Design review of the part built by this model. Coordinates are the model's own, in mm. Face numbers are marked on the shaded views. A direction names the side the tool comes from. Give positions to 0.01 mm unless a question says otherwise; leave off trailing zeros. Write each loop counter-clockwise with the first axis right and the second up, starting at its lowest first coordinate (ties: lowest second). Pieces come first, ordered by that corner, then holes.
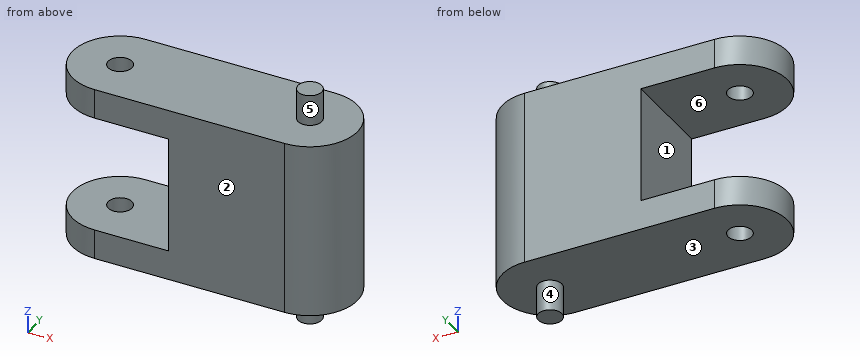
```python
from build123d import *

# Parameters (mm, degrees)
CROQUIS1_R                    = 9.977
SALIENTE_EXTRUIR9_DEPTH       = 148
SALIENTE_EXTRUIR10_DEPTH      = 26
SALIENTE_EXTRUIR10_DEPTH_BACK = 174
CROQUIS8_R                    = 9.977
CROQUIS9_W                    = 114.38894851
CROQUIS9_H                    = 98
CORTAR_EXTRUIR2_DEPTH         = 131


with BuildPart() as part:
    # Croquis1 → Saliente-Extruir9 (new body)
    with BuildSketch(Plane.XY):
        with BuildLine():
            Line((0, 40), (160, 40))
            ThreePointArc((160, 40), (200, 0), (160, -40))
            Line((160, -40), (0, -40))
            ThreePointArc((0, -40), (-40, 0), (0, 40))
        make_face()
        Circle(CROQUIS1_R, mode=Mode.SUBTRACT)
    extrude(amount=SALIENTE_EXTRUIR9_DEPTH)

    # Croquis8 → Saliente-Extruir10 (add, two sides: drawn at the far end of the back side and taken through both)
    with BuildSketch(Plane(origin=(0, 0, 0), x_dir=(-1, 0, 0), z_dir=(0, 0, -1)).offset(-SALIENTE_EXTRUIR10_DEPTH_BACK)):
        with Locations((-160, 0)):
            Circle(CROQUIS8_R)
    extrude(amount=SALIENTE_EXTRUIR10_DEPTH + SALIENTE_EXTRUIR10_DEPTH_BACK)

    # Croquis9 → Cortar-Extruir2 (cut)
    with BuildSketch(Plane(origin=(0, 40, 0), x_dir=(1, 0, 0), z_dir=(0, 1, 0))):
        with Locations((4.810807807, -74)):
            Rectangle(CROQUIS9_W, CROQUIS9_H)
    extrude(amount=-CORTAR_EXTRUIR2_DEPTH, mode=Mode.SUBTRACT)


solid = part.part
```
(1) Tool access review of the marked faces 4, 5 and 6: name each direction out of +Z, -Z, +X, -X, +Y, -Y from which nothing blocks a thin tool from reaching the whole face with its end or side.
Resolved:
face 4: -Z
face 5: +Z
face 6: -X, +Y, -Y
(2) Consider section C-C, the plane x = 79. Give the boundary of the cut face in (y, z), then the cut area to 3 significant figures.
Resolved:
outline: (-40, 0) - (40, 0) - (40, 148) - (-40, 148) - close
area: 11,800 mm2
(3) Mouldability with a two-part tool opening along Z and no side actions: class the marked faces 1, 2 and 3 as pulls with the +Z half, pulls with the -Z half, needs draft (parallel to the pull), parting line crosses it, or undercut.
Resolved:
face 1: undercut
face 2: needs draft
face 3: pulls with the -Z half
(4) To check wall thickness, follow L1, parallel to Y at x = 0, z = 141.5; L2, parallel to Z at x = 57, y = -3.5; L3, parallel to X at y = 0, z = 10.5. State the ranges of each line that lie inside material, in increasing order.
Resolved:
L1: y = -40 to -9.98, 9.98 to 40
L2: z = 0 to 25, 123 to 148
L3: x = -40 to -9.98, 9.98 to 200
(5) Consider section D-D, the plane y = -16. Give the boundary of the cut face in (x, z), then the cut area to 3 significant figures.
Resolved:
outline: (-36.66, 0) - (196.66, 0) - (196.66, 148) - (-36.66, 148) - (-36.66, 123) - (62.01, 123) - (62.01, 25) - (-36.66, 25) - close
area: 24,900 mm2
(6) Consider section A-A, the plane y = 0. Give the boundary of the cut face in (x, z), then the cut area to 3 significant figures.
Resolved:
outline: (-40, 0) - (-9.98, 0) - (-9.98, 25) - (-40, 25) - close; (-40, 123) - (-9.98, 123) - (-9.98, 148) - (-40, 148) - close; (9.98, 0) - (150.02, 0) - (150.02, -26) - (169.98, -26) - (169.98, 0) - (200, 0) - (200, 148) - (169.98, 148) - (169.98, 174) - (150.02, 174) - (150.02, 148) - (9.98, 148) - (9.98, 123) - (62.01, 123) - (62.01, 25) - (9.98, 25) - close
area: 25,600 mm2
(7) Consider section B-B, the plane x = 13. Give the boundary of the cut face in (y, z).
Resolved:
outline: (-40, 0) - (40, 0) - (40, 25) - (-40, 25) - close; (-40, 123) - (40, 123) - (40, 148) - (-40, 148) - close
(8) Clearance check with flat-ended pins moving along their axes: P1, Ø2, axis at x = -8, z = 5.5, coming from the -Y side; P2, Ø24, axis at x = -8, y = 15, coming from the -Z side; P3, Ø23, axis at x = 0, y = 0, coming from the +Z side. State where each tip first meets the part, or that it passes through.
Resolved:
P1: stops at y = -39.38
P2: stops at z = 0
P3: stops at z = 148
